Could you check a few things on this model? Use its own coordinates, in mm. A direction names the side the tool comes from. Coordinates: 2 decimals unless noted, no trailing zeros. Loops run counter-clockwise (first coordinate to the right, second up) from the corner with the lowest first, then second, coordinate; pieces in that order, holes last. Notation, with made-up numbers: M 4,66 L 40,66 A30 ccw 40,96 Z; hole C 43.25,35 d11. An arc over 180 degrees is marked long. Return JSON: item names as keys, results as strings. Group by question number.
from build123d import *

# Parameters (mm, degrees)
BOSS_EXTRUDE1_DEPTH = 12
CUT_EXTRUDE1_REACH  = 22
BOSS_EXTRUDE2_DEPTH = 6
SKETCH4_R           = 2
BOSS_EXTRUDE3_DEPTH = 3.5


with BuildPart() as part:
    # Sketch1 → Boss-Extrude1 (new body)
    with BuildSketch(Plane.XY):
        Polygon((-16, 10), (-16, 8), (-11, 8), (-11, -10), (11, -10), (11, 8), (16, 8), (16, 10), (11, 10), (11, 11), (-11, 11), (-11, 10), align=None)
    extrude(amount=BOSS_EXTRUDE1_DEPTH)

    # Sketch2 → Cut-Extrude1 (cut, up to next)
    with BuildSketch(Plane(origin=(0, 10, 0), x_dir=(1, 0, 0), z_dir=(0, 1, 0)), mode=Mode.PRIVATE) as cut_extrude1_sk1:
        with BuildLine():
            Line((-16, -6), (-14.871798323, -6))
            ThreePointArc((-14.871798323, -6), (-12.900501279, -6.237869823), (-14.871798323, -6.475739646))
            Line((-14.871798323, -6.475739646), (-16, -6.475739646))
            Line((-16, -6.475739646), (-16, -6))
        make_face()
    cut_extrude1_tool1 = extrude(cut_extrude1_sk1.sketch, amount=-CUT_EXTRUDE1_REACH, mode=Mode.PRIVATE) & part.part
    add(cut_extrude1_tool1.solids().sort_by_distance((-14.122654, 10, 6.23787))[0], mode=Mode.SUBTRACT)
    # Sketch2 → Cut-Extrude1 (cut, up to next)
    with BuildSketch(Plane(origin=(0, 10, 0), x_dir=(1, 0, 0), z_dir=(0, 1, 0)), mode=Mode.PRIVATE) as cut_extrude1_sk2:
        with BuildLine():
            Line((16, -6.237869823), (14.871798323, -6.237869823))
            ThreePointArc((14.871798323, -6.237869823), (12.900501279, -6), (14.871798323, -5.762130177))
            Line((14.871798323, -5.762130177), (16, -5.762130177))
            Line((16, -5.762130177), (16, -6.237869823))
        make_face()
    cut_extrude1_tool2 = extrude(cut_extrude1_sk2.sketch, amount=-CUT_EXTRUDE1_REACH, mode=Mode.PRIVATE) & part.part
    add(cut_extrude1_tool2.solids().sort_by_distance((14.122654, 10, 6))[0], mode=Mode.SUBTRACT)

    # Sketch3 → Boss-Extrude2 (add)
    with BuildSketch(Plane(origin=(0, 11, 0), x_dir=(1, 0, 0), z_dir=(0, 1, 0))):
        with BuildLine():
            ThreePointArc((-0.34375, -8.72843104), (11, -6), (-0.34375, -3.27156896))
            ThreePointArc((-0.34375, -3.27156896), (-2.75, -6), (-0.34375, -8.72843104))
        make_face()
    extrude(amount=BOSS_EXTRUDE2_DEPTH)

    # Sketch4 → Boss-Extrude3 (add)
    with BuildSketch(Plane(origin=(0, 17, 0), x_dir=(1, 0, 0), z_dir=(0, 1, 0))):
        with Locations((5, -6)):
            Circle(SKETCH4_R)
    extrude(amount=BOSS_EXTRUDE3_DEPTH)


solid = part.part
(1) Will these pins go through, and if not, where does the flat tip stop? P1, Ø1.8, axis at x = -13.9, z = 6.24, coming from the +Y side; P2, Ø0.8, axis at y = 10.5, z = 5, coming from the +X side; P3, Ø1.8, axis at x = 8, z = 9, coming from the +Y side; P4, Ø2.5, axis at x = 13.9, z = 6, coming from the -Y side.
(2) We'd pull the mould along Z, two halves only. Please class faces 6 (the face through (15.4, 9, 6.238)), 7 (the face through (0, -10, 6)), 8 (the face through (-2.75, 13.96, 5.94)): +Z half, -Z half, draft (parallel to the pull), parting line (faces both ways), or undercut.
(3) Imagine slicing it at D-D, the plane y = -5. Write out the boundary of the cut face in (x, z), then the cut area to 3 significant figures.
(4) For faces 1 (the face through (-12, 10, 6)), 2 (the face through (11, 14, 6)), 3 (the face through (15.4, 9, 5.762)), 4 (the face through (-12, 8, 6)), 5 (the face through (-15.4, 9, 6.476)), which set-ups out of +Z, -Z, +X, -X, +Y, -Y let a thin tool reach every point of the face, with its end or its side?
(5) Imagine slicing it at C-C, the plane x = -12. Write out the boundary of the cut face in (y, z).
(6) If I drill on L1, parallel to Y at x = -1.5, z = 2; L2, parallel to Y at x = 8.5, z = 10; L3, parallel to X at y = -6, z = 2.25, over which ranges is the centre line in solid material (lowest first)? Write a range as [from, to].
(7) Imagine slicing it at B-B, the plane y = 16. Write out the boundary of the cut face in (x, z).
(8) Imagine slicing it at A-A, the plane z = 10. Write out the boundary of the cut face in (x, y).
Checks:
{
 "1": {"P1": "through", "P2": "x = 11", "P3": "y = 17", "P4": "y = 8"},
 "2": {"face 6": "undercut", "face 7": "draft", "face 8": "parting line"},
 "3": {"outline": "M -11,0 L 11,0 L 11,12 L -11,12 Z", "area": "264 mm²"},
 "4": {"face 1": "+Z, -Z, -X, +Y", "face 2": "+Y", "face 3": "+X, +Y, -Y", "face 4": "+Z, -Z, -X, -Y", "face 5": "-X, +Y, -Y"},
 "5": {"outline": "M 8,0 L 10,0 L 10,12 L 8,12 Z"},
 "6": {"L1": "[-10, 11]", "L2": "[-10, 17]", "L3": "[-11, 11]"},
 "7": {"outline": "M -0.34,3.27 A6 ccw long -0.34,8.73 A2.75 ccw Z"},
 "8": {"outline": "M -16,8 L -11,8 L -11,-10 L 11,-10 L 11,8 L 16,8 L 16,10 L 11,10 L 11,11 L 9.47,11 L 9.47,17 L 0.53,17 L 0.53,11 L -11,11 L -11,10 L -16,10 Z"}
}
